Part model, mm, in its own coordinate system. Face numbers are marked on the shaded views. A direction names the side the tool comes from. Give positions to 0.01 mm unless a question says otherwise; leave off trailing zeros. Order: outer loops, then holes, each group sorted by start corner. A loop starts at its lowest first (then second) coordinate and runs counter-clockwise, first axis right, second up. Notation, with made-up numbers: M 49,49 L 94,49 A19 ccw 94,71 Z; hole C -30,41 d1. An arc over 180 degrees is marked long. One line per question, with ' | ' between items.
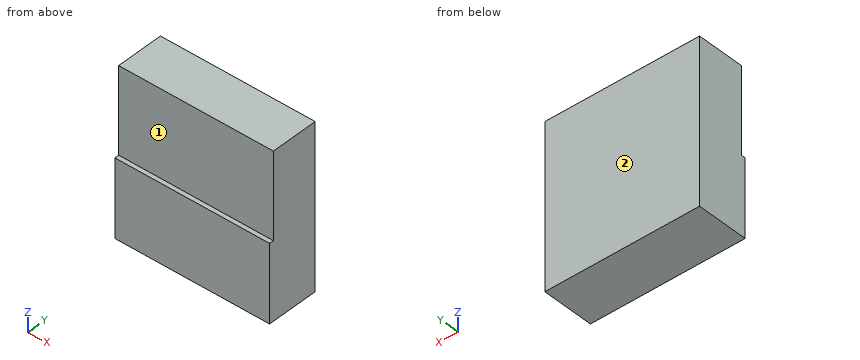
```python
from build123d import *

# Parameters (mm, degrees)
F0_W     = 457.2
F0_H     = 457.2
F1_DEPTH = 152.4
F2_W     = 457.2
F2_H     = 228.6
F3_DEPTH = 12.7
F4_W     = 457.2
F4_H     = 139.7
F5_DEPTH = 25.4


with BuildPart() as f1:
    # F0 (on Front) → F1 (new body)
    with BuildSketch(Plane.XZ):
        Rectangle(F0_W, F0_H)
    extrude(amount=F1_DEPTH)

    # F2 (on face) → F3 (cut)
    with BuildSketch(Plane.XZ.offset(152.4)):
        with Locations((0, 114.3)):
            Rectangle(F2_W, F2_H)
    extrude(amount=-F3_DEPTH, mode=Mode.SUBTRACT)

    # F4 (on face) → F5 (join)
    with BuildSketch(Plane.XY.offset(228.6)):
        with Locations((0, -69.85)):
            Rectangle(F4_W, F4_H)
    extrude(amount=F5_DEPTH)


solid = f1.part
```
1. Slice it at B-B on z = 66.5. Give the cut face in (x, y), then the cut area to 3 significant figures.
Worked out:
outline: M -228.6,-139.7 L 228.6,-139.7 L 228.6,0 L -228.6,0 Z | area: 63,900 mm2
2. Slice it at A-A on x = -186. Give the cut face in (y, z), then the cut area to 3 significant figures.
Worked out:
outline: M -152.4,-228.6 L 0,-228.6 L 0,254 L -139.7,254 L -139.7,0 L -152.4,0 Z | area: 70,300 mm2
3. Tool access for the marked faces 1 and 2: list every direction of +Z, -Z, +X, -X, +Y, -Y with a clear straight run to the whole face (end or side of a thin tool).
Worked out:
face 1: +Z, +X, -X, -Y | face 2: +Z, -Z, +X, -X, +Y
4. Drop a flat-ended pin along its axis: pin 1 (4 mm diameter, centred on x = 0, y = -145, fed in from +Z). Give the stop position or say it passes through.
Worked out:
pin 1: stops at z = 0
5. Probe L1, parallel to Z at x = -48, y = -143; L2, parallel to Y at x = 110, z = 2. List the from-to ranges inside material, lowest first. Write a range as from..to.
Worked out:
L1: z = -228.6..0 | L2: y = -139.7..0
